Can you work these out from the drawing? Everything is in mm from the part's minimum corner. A direction names the side the tool comes from. Give positions to 0.01 mm unless a question says otherwise; leave off trailing zeros. Order: outer loops, then holes, each group sorted by start corner. A loop starts at its lowest first (then second) coordinate and runs counter-clockwise, first axis right, second up. Notation, with made-up numbers: M -22,-34.75 L 14,-34.75 A23 cw 14,-21.75 Z; hole C 55.5,52.25 d6. An arc over 180 degrees is marked long. Answer as a JSON object with one key per item and string values.
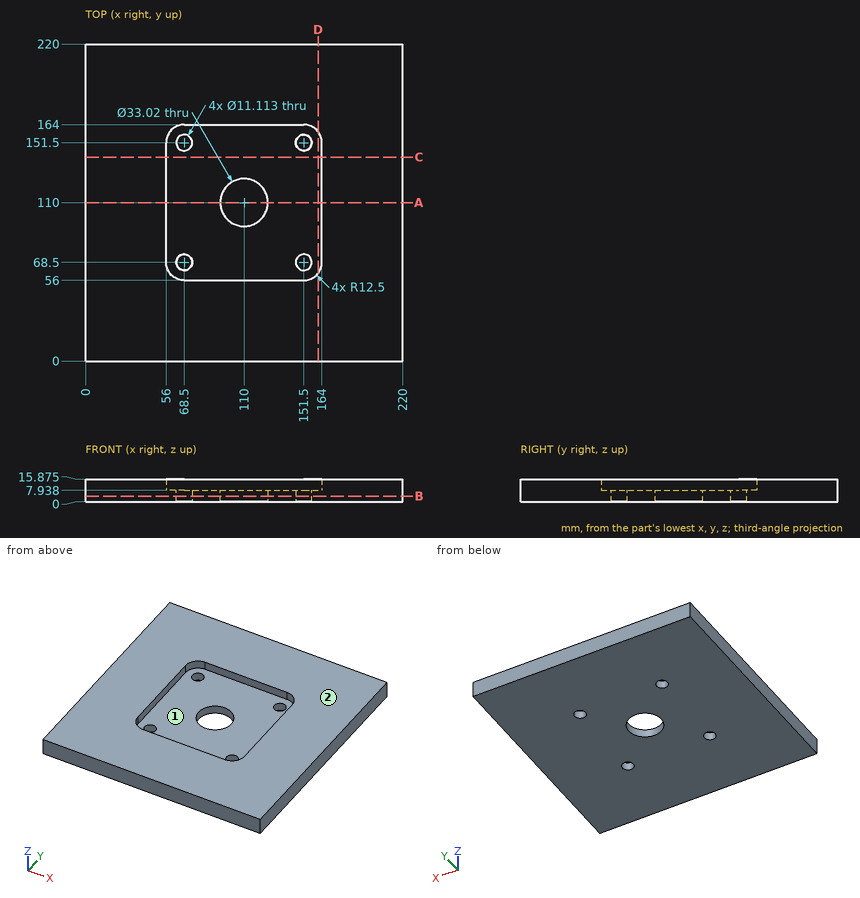
1) I'm going to push a flat-ended pin straight in: pin 1 Ø2 at (x, y) = (137, 133.5) entering from +Z. Where does the tip first touch, or does it pass through?
Results found:
{"pin 1": "stops at z = 7.94"}
2) I want a section at D-D on x = 161.5. Write out the boundary of the cut face in (y, z) (1 decimal).
Results found:
{"outline": "M 0,0 L 220,0 L 220,15.9 L 159,15.9 L 159,7.9 L 61,7.9 L 61,15.9 L 0,15.9 Z"}
3) I want a section at B-B on z = 4. Write out the boundary of the cut face in (x, y).
Results found:
{"outline": "M 0,0 L 220,0 L 220,220 L 0,220 Z; hole C 68.5,68.5 d11.11; hole C 68.5,151.5 d11.11; hole C 110,110 d33.02; hole C 151.5,68.5 d11.11; hole C 151.5,151.5 d11.11"}
4) For the marked faces 1 and 2, which set-ups out of +Z, -Z, +X, -X, +Y, -Y let a thin tool reach every point of the face, with its end or its side?
Results found:
{"face 1": "+Z", "face 2": "+Z, +X, -X, +Y, -Y"}
5) I need wall thicknesses on L1, parallel to Y at x = 151.5, z = 6; L2, parallel to X at y = 133, z = 13. Which ranges of each line are inside material? Lowest first, please.
Results found:
{"L1": "y = 0 to 62.94, 74.06 to 145.94, 157.06 to 220", "L2": "x = 0 to 56, 164 to 220"}
6) I want a section at C-C on y = 141.5. Write out the boundary of the cut face in (x, z) (1 decimal).
Results found:
{"outline": "M 0,0 L 220,0 L 220,15.9 L 164,15.9 L 164,7.9 L 56,7.9 L 56,15.9 L 0,15.9 Z"}
7) I want a section at A-A on y = 110. Write out the boundary of the cut face in (x, z) (1 decimal).
Results found:
{"outline": "M 0,0 L 93.5,0 L 93.5,7.9 L 56,7.9 L 56,15.9 L 0,15.9 Z; M 126.5,0 L 220,0 L 220,15.9 L 164,15.9 L 164,7.9 L 126.5,7.9 Z"}
